Can you work these out from the model? Positions are in its coordinate system, mm. Face numbers are marked on the shaded views. Round coordinates to 2 decimals unless told otherwise and drop trailing zeros. Write each loop counter-clockwise with the first axis right and the second up, starting at its lowest first coordinate (ties: lowest second). Pieces come first, ordered by that corner, then holes. Notation, with made-up numbers: M 63.25,2 L 120.25,2 A18 ccw 120.25,8 Z; hole C -17,41 d1. An arc over 180 degrees is marked long. Answer as a JSON object with one key per item and string values. Group by question number.
1) Suppose I cut it at C-C, the plane y = -12. Write out the boundary of the cut face in (x, z), and give its area (3 significant figures).
2) I'm going to push flat-ended pins straight in: pin 1 Ø3 at (y, z) = (8, 8) entering from -X; pin 2 Ø3 at (x, z) = (21, 0.5) entering from -Y; pin 3 Ø4 at (y, z) = (1, -7) entering from +X. Where does each tip first touch, or does it pass through?
3) Suppose I cut it at B-B, the plane x = 4. Write out the boundary of the cut face in (y, z), and give its area (3 significant figures).
4) Please list where these lines run through material, in increasing order: L1, parallel to X at y = -31.5, z = 0; L2, parallel to Y at x = 0, z = 3; L3, parallel to X at y = -26.5, z = -0.5. Write a range as [from, to].
5) Suppose I cut it at A-A, the plane z = 0. Write out the boundary of the cut face in (x, y), and give its area (3 significant figures).
6) If we mould it in two halves opening along X, with no side actions, what happens to the marked faces 1, 2, 3 and 4? For each: +X half, -X half, draft (parallel to the pull), parting line (faces both ways), or undercut.
from build123d import *

# Parameters (mm, degrees)
EXTRUDE_1_DEPTH = 30
FILLET_1_R      = 3
SKETCH_2_R      = 3
SKETCH_2_R_2    = 4.5
EXTRUDE_2_DEPTH = 3


with BuildPart() as part:
    # 草图1 → 凸台-拉伸1 (new, symmetric)
    with BuildSketch(Plane(origin=(0, 0, 0), x_dir=(1, 0, 0), z_dir=(0, 1, 0))):
        with BuildLine():
            Line((-20, 10), (20, 10))
            ThreePointArc((20, 10), (30, 0), (20, -10))
            Line((20, -10), (-20, -10))
            ThreePointArc((-20, -10), (-30, 0), (-20, 10))
        make_face()
    extrude(amount=EXTRUDE_1_DEPTH, both=True)

    # 圆角1
    fillet_1_edges = [part.edges().sort_by_distance(p)[0] for p in [
        (30, 30, 0),
        (0, 30, -10),
        (-30, 30, 0),
        (0, 30, 10),
    ]]
    fillet(fillet_1_edges, radius=FILLET_1_R)

    # 草图2 → 凸台-拉伸2 (add)
    # profile 1 of 2: a face of its own
    with BuildSketch(Plane.XZ.offset(30)):
        with Locations(Location((-20, 0, 0), (0, 0, 90))):
            Circle(SKETCH_2_R)
    # profile 2 of 2: a face of its own
    with BuildSketch(Plane.XZ.offset(30)):
        with Locations(Location((20, 0, 0), (0, 0, 90))):
            Circle(SKETCH_2_R_2)
        with Locations(Location((20, 0, 0), (0, 0, 270))):
            Circle(SKETCH_2_R, mode=Mode.SUBTRACT)
    extrude(amount=EXTRUDE_2_DEPTH)


solid = part.part
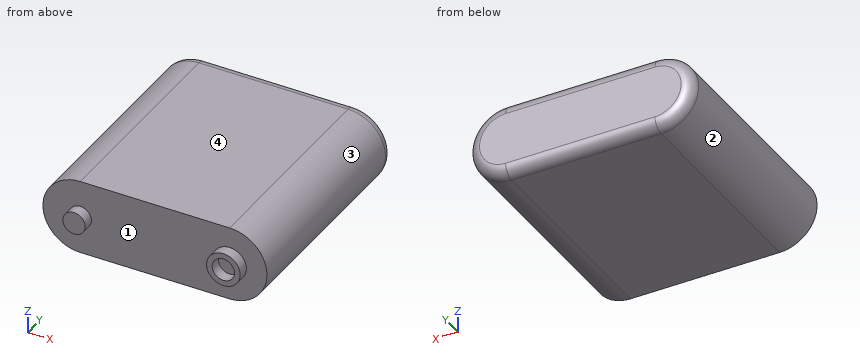
Results:
{
 "1": {"outline": "M -20,-10 L 20,-10 A10 ccw 20,10 L -20,10 A10 ccw Z", "area": "1,110 mm^2"},
 "2": {"pin 1": "x = -27.6", "pin 2": "y = -30", "pin 3": "x = 28.66"},
 "3": {"outline": "M -30,-10 L 27,-10 A3 ccw 30,-7 L 30,7 A3 ccw 27,10 L -30,10 Z", "area": "1,200 mm^2"},
 "4": {"L1": "[-23, -17], [15.5, 17], [23, 24.5]", "L2": "[-30, 30]", "L3": "[-29.99, 29.99]"},
 "5": {"outline": "M -30,-30 L -23,-30 L -23,-33 L -17,-33 L -17,-30 L 15.5,-30 L 15.5,-33 L 17,-33 L 17,-30 L 23,-30 L 23,-33 L 24.5,-33 L 24.5,-30 L 30,-30 L 30,27 A3 ccw 27,30 L -27,30 A3 ccw -30,27 Z", "area": "3,620 mm^2"},
 "6": {"face 1": "undercut", "face 2": "-X half", "face 3": "+X half", "face 4": "draft"}
}
